Input: part model. Units: mm. Frame: model coordinates. Face numbers are marked on the shaded views. A direction names the side the tool comes from. Coordinates: 2 decimals unless noted, no trailing zeros. Loops run counter-clockwise (first coordinate to the right, second up) from the corner with the lowest first, then second, coordinate; pieces in that order, holes last. Notation, with made-up numbers: (56.25, 81) - (67.25, 81) arc R16 cw to (67.25, 111) - close; hole circle Ø5 at (25, 4). An arc over 180 degrees is marked (long way). Write item = value, one per line. Start each with the question number.
from build123d import *

# Parameters (mm, degrees)
F0_R     = 1
F1_DEPTH = 15
F3_DEPTH = 23
F4_W     = 30
F4_H     = 15
F5_DEPTH = 3
F6_R     = 3


with BuildPart() as f1:
    # F0 (on Top) → F1 (new body)
    with BuildSketch(Plane.XY):
        Polygon((-10, 10), (-10, -10), (10, -10), (10, 7.8278025612), (10, 10), align=None)
        with Locations((7.3302448727, -7.8278025612)):
            Circle(F0_R, mode=Mode.SUBTRACT)
        with BuildLine():
            ThreePointArc((-3.9921798557, 0.25), (0.1250611397, 3.9980444859), (4, 0))
            ThreePointArc((4, 0), (0.1250611397, -3.9980444859), (-3.9921798557, -0.25))
            Line((-3.9921798557, -0.25), (-8.3, -0.25))
            Line((-8.3, -0.25), (-8.3, 0))
            Line((-8.3, 0), (-8.3, 0.25))
            Line((-8.3, 0.25), (-3.9921798557, 0.25))
        make_face(mode=Mode.SUBTRACT)
        with Locations((7.3302448727, 7.8278025612)):
            Circle(F0_R, mode=Mode.SUBTRACT)
        Polygon((10, 7.8278025612), (10, -10), (30, -10), (30, 10), (10, 10), align=None)
        with Locations((27.6660211384, -7.8278025612)):
            Circle(F0_R, mode=Mode.SUBTRACT)
        with BuildLine():
            ThreePointArc((28.6660211384, 7.8278025612), (27.6660211384, 6.8278025612), (26.6660211384, 7.8278025612))
            ThreePointArc((26.6660211384, 7.8278025612), (27.6660211384, 8.8278025612), (28.6660211384, 7.8278025612))
        make_face(mode=Mode.SUBTRACT)
        with Locations((7.3302448727, 7.8278025612)):
            Circle(F0_R)
        with BuildLine():
            ThreePointArc((28.6660211384, 7.8278025612), (27.6660211384, 8.8278025612), (26.6660211384, 7.8278025612))
            ThreePointArc((26.6660211384, 7.8278025612), (27.6660211384, 6.8278025612), (28.6660211384, 7.8278025612))
        make_face()
    extrude(amount=F1_DEPTH)

    # F2 (on face) → F3 (cut)
    with BuildSketch(Plane.YZ.offset(30)):
        Polygon((-5.15, 12.65), (-5.15, 7.5), (-5.15, 2.35), (5.15, 2.35), (5.15, 12.65), align=None)
    extrude(amount=-F3_DEPTH, mode=Mode.SUBTRACT)

    # F4 (on face) → F5 (join)
    with BuildSketch(Plane(origin=(0, 10, 0), x_dir=(-1, 0, 0), z_dir=(0, 1, 0))):
        with BuildLine():
            Line((-30, 37), (-30, 26.4))
            Line((-30, 26.4), (-20.15, 26.4))
            ThreePointArc((-20.15, 26.4), (-18.6415999231, 30.0415999231), (-15, 31.55))
            Line((-15, 31.55), (-15, 37))
            Line((-15, 37), (-30, 37))
        make_face()
        with Locations((-15, 7.5)):
            Rectangle(F4_W, F4_H)
        with BuildLine():
            Line((-30, 26.4), (-30, 15))
            Line((-30, 15), (0, 15))
            Line((0, 15), (0, 37))
            Line((0, 37), (-15, 37))
            Line((-15, 37), (-15, 31.55))
            ThreePointArc((-15, 31.55), (-11.3584000769, 30.0415999231), (-9.85, 26.4))
            ThreePointArc((-9.85, 26.4), (-15, 21.25), (-20.15, 26.4))
            Line((-20.15, 26.4), (-30, 26.4))
        make_face()
    extrude(amount=-F5_DEPTH)

    # F6
    f6_edges = [f1.edges().sort_by_distance(p)[0] for p in [
        (30, 8.5, 37),
        (0, 8.5, 37),
    ]]
    fillet(f6_edges, radius=F6_R)


solid = f1.part
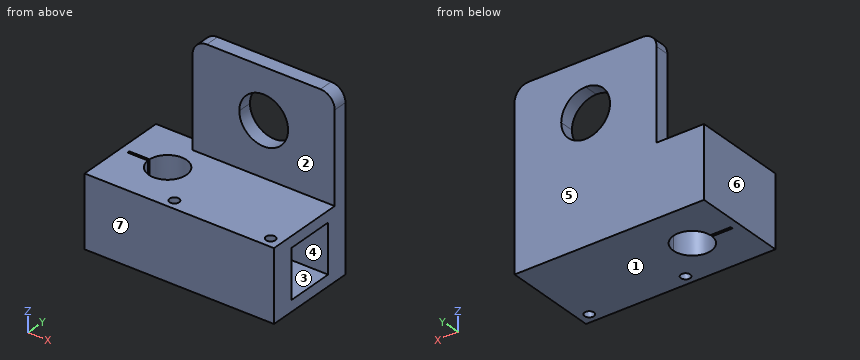
Item 1: Pull-direction query (Y, two-part tool) for the marked faces 4, 5, 6 and 7; classes: pulls with the +Y half, pulls with the -Y half, needs draft (parallel to the pull), parting line crosses it, or undercut.
Item 2: Cut plane B-B on y = 2. Return loops of the section in (x, z).
Item 3: Pin query (flat end, axial travel): pin 1 (3 mm diameter, centred on y = 0.5, z = 8, fed in from +X); pin 2 (8 mm diameter, centred on x = 16, y = -0.5, fed in from +Z); pin 3 (3.5 mm diameter, centred on y = 9, z = 24.5, fed in from -X). Return the tip coordinate at first contact, or that it passes through.
Item 4: Cut plane C-C on y = 4.5. Return loops of the section in (x, z).
Item 5: Cut plane D-D on z = 30. Return loops of the section in (x, y), plus the area to 3 significant figures.
Item 6: Cut plane A-A on x = 18.5. Return loops of the section in (y, z), plus the area to 3 significant figures.
Item 7: Ray query, line 1 (Y direction, x = 14.5, z = 11); line 2 (X direction, y = -8, z = 7); line 3 (Z direction, x = 16.5, y = 4.75). Return the intervals inside material, ascending.
Item 8: Access query for the marked faces 1, 2 and 3. Directions: +Z, -Z, +X, -X, +Y, -Y. A direction counts if a zero-diameter tool reaches every point of the face in a straight line with its end or side. Return the directions, or none.
Recorded:
q1.face_4 = undercut
q1.face_5 = pulls with the +Y half
q1.face_6 = needs draft
q1.face_7 = pulls with the -Y half
q2.outline = (-10, 0) - (-3.46, 0) - (-3.46, 15) - (-10, 15) - close; (3.46, 0) - (30, 0) - (30, 2.35) - (7, 2.35) - (7, 12.65) - (30, 12.65) - (30, 15) - (3.46, 15) - close
q3.pin_1 = 7
q3.pin_2 = 15
q3.pin_3 = 0
q4.outline = (-10, 0) - (30, 0) - (30, 2.35) - (7, 2.35) - (7, 12.65) - (30, 12.65) - (30, 15) - (-10, 15) - close
q5.outline = (0, 7) - (11.32, 7) - (11.32, 10) - (0, 10) - close; (18.68, 7) - (30, 7) - (30, 10) - (18.68, 10) - close
q5.area = 67.9 mm²
q6.outline = (-10, 0) - (10, 0) - (10, 22.62) - (7, 22.62) - (7, 15) - (-10, 15) - close; (7, 30.18) - (10, 30.18) - (10, 37) - (7, 37) - close; hole (-5.15, 2.35) - (5.15, 2.35) - (5.15, 12.65) - (-5.15, 12.65) - close
q6.area = 237 mm²
q7.line_1 = -10 to -5.15, 5.15 to 10
q7.line_2 = -10 to 6.35, 8.32 to 26.68, 28.65 to 30
q7.line_3 = 0 to 2.35, 12.65 to 15
q8.face_1 = -Z, +X, -X, +Y, -Y
q8.face_2 = +Z, +X, -X, -Y
q8.face_3 = +X
